```python
from build123d import *

# Parameters (mm, degrees)
SKETCH1_R           = 1.5
SKETCH1_R_2         = 2
SKETCH1_R_3         = 8
BOSS_EXTRUDE1_DEPTH = 5


with BuildPart() as part:
    # Sketch1 → Boss-Extrude1 (new body)
    with BuildSketch(Plane.XY):
        with BuildLine():
            Line((-15, 70), (-29.20308374, 7.195041803))
            ThreePointArc((-29.20308374, 7.195041803), (-0.112734709, -30.136506004), (28.977614322, 7.195041803))
            Line((28.977614322, 7.195041803), (15, 70))
            Line((15, 70), (-15, 70))
        make_face()
        with Locations((-12.5, -21.650635095)):
            Circle(SKETCH1_R, mode=Mode.SUBTRACT)
        with Locations((0, -17.5)):
            Circle(SKETCH1_R_2, mode=Mode.SUBTRACT)
        with Locations((-25, 0)):
            Circle(SKETCH1_R, mode=Mode.SUBTRACT)
        with Locations((-17.5, 0)):
            Circle(SKETCH1_R_2, mode=Mode.SUBTRACT)
        with Locations((-12.5, 21.650635095)):
            Circle(SKETCH1_R, mode=Mode.SUBTRACT)
        with Locations((12.5, -21.650635095)):
            Circle(SKETCH1_R, mode=Mode.SUBTRACT)
        Circle(SKETCH1_R_3, mode=Mode.SUBTRACT)
        with BuildLine():
            ThreePointArc((0, 15.5), (-2, 17.5), (0, 19.5))
            ThreePointArc((0, 19.5), (2, 17.5), (0, 15.5))
        make_face(mode=Mode.SUBTRACT)
        with Locations((12.5, 21.650635095)):
            Circle(SKETCH1_R, mode=Mode.SUBTRACT)
        with Locations((17.5, 0)):
            Circle(SKETCH1_R_2, mode=Mode.SUBTRACT)
        with Locations((25, 0)):
            Circle(SKETCH1_R, mode=Mode.SUBTRACT)
        with Locations((-7.5, 45)):
            Circle(SKETCH1_R_2, mode=Mode.SUBTRACT)
        with Locations((-7.5, 55)):
            Circle(SKETCH1_R_2, mode=Mode.SUBTRACT)
        with Locations((-7.5, 65)):
            Circle(SKETCH1_R_2, mode=Mode.SUBTRACT)
        with Locations((7.5, 65)):
            Circle(SKETCH1_R_2, mode=Mode.SUBTRACT)
        with Locations((7.5, 55)):
            Circle(SKETCH1_R_2, mode=Mode.SUBTRACT)
        with Locations((7.5, 45)):
            Circle(SKETCH1_R_2, mode=Mode.SUBTRACT)
    extrude(amount=BOSS_EXTRUDE1_DEPTH)


solid = part.part
```
The listing builds one solid part. Answer for the finished solid, in the listing's coordinates (mm). Round coordinates to 2 decimals unless told otherwise and drop trailing zeros. Order: outer loops, then holes, each group sorted by start corner. A loop starts at its lowest first (then second) coordinate and runs counter-clockwise, first axis right, second up. Notation, with made-up numbers: (3, 83.25) -> (40, 83.25) arc R26 cw to (40, 99.25) -> close; hole circle Ø10 at (-36.75, 28.5). An arc over 180 degrees is marked (long way). Answer as CSV lines item,"result". Start each with the question number.
(1) The part is cut by section A-A (x = 17.5). Determine the outline of the cut face in (y, z), then the cut area to 3 significant figures.
(2) For a pull along Y with two mould halves and no side action, classify faces 1 (the face through (-1.73, -7.81, 2.46)), 2 (the face through (-1, 21, 5)), 3 (the face through (0, 70, 2)) as +Y half, -Y half, draft (parallel to the pull), parting line (faces both ways), or undercut.
(3) Find the intervals of material crossed by probe 1 along Y at (x, z) = (-7, 1.35); probe 2 along Y at (x, z) = (12.5, 1.65); probe 3 along Y at (x, z) = (13, 2.1), in increasing order. Write a range as from..to.
(4) The part is cut by section C-C (y = 0). Determine the outline of the cut face in (x, z).
(5) A flat-ended cylindrical pin translates along its axis: pin 1 Ø1.5 at (y, z) = (28, 1) entering from +X. Find the tip coordinate at first contact, or state that the pin passes through.
(6) The part is cut by section D-D (x = 0). Determine the outline of the cut face in (y, z), then the cut area to 3 significant figures.
(7) The part is cut by section B-B (y = 45). Determine the outline of the cut face in (x, z).
Evaluation:
1,outline,"(-24.42, 0) -> (-2, 0) -> (-2, 5) -> (-24.42, 5) -> close; (2, 0) -> (58.77, 0) -> (58.77, 5) -> (2, 5) -> close"
1,area,"396 mm²"
2,face 1,"undercut"
2,face 2,"draft"
2,face 3,"+Y half"
3,probe 1,"-29.34..-3.87, 3.87..43.06, 46.94..53.06, 56.94..63.06, 66.94..70"
3,probe 2,"-27.36..-23.15, -20.15..20.15, 23.15..70"
3,probe 3,"-27.12..-23.06, -20.24..20.24, 23.06..70"
4,outline,"(-30.11, 0) -> (-26.5, 0) -> (-26.5, 5) -> (-30.11, 5) -> close; (-23.5, 0) -> (-19.5, 0) -> (-19.5, 5) -> (-23.5, 5) -> close; (-15.5, 0) -> (-8, 0) -> (-8, 5) -> (-15.5, 5) -> close; (8, 0) -> (15.5, 0) -> (15.5, 5) -> (8, 5) -> close; (19.5, 0) -> (23.5, 0) -> (23.5, 5) -> (19.5, 5) -> close; (26.5, 0) -> (29.89, 0) -> (29.89, 5) -> (26.5, 5) -> close"
5,pin 1,"x = 24.51"
6,outline,"(-30.14, 0) -> (-19.5, 0) -> (-19.5, 5) -> (-30.14, 5) -> close; (-15.5, 0) -> (-8, 0) -> (-8, 5) -> (-15.5, 5) -> close; (8, 0) -> (15.5, 0) -> (15.5, 5) -> (8, 5) -> close; (19.5, 0) -> (70, 0) -> (70, 5) -> (19.5, 5) -> close"
6,area,"381 mm²"
7,outline,"(-20.65, 0) -> (-9.5, 0) -> (-9.5, 5) -> (-20.65, 5) -> close; (-5.5, 0) -> (5.5, 0) -> (5.5, 5) -> (-5.5, 5) -> close; (9.5, 0) -> (20.56, 0) -> (20.56, 5) -> (9.5, 5) -> close"
